The model under review builds one solid part; all positions refer to its coordinate system, in mm. A direction names the side the tool comes from. Coordinates: 2 decimals unless noted, no trailing zeros. Loops run counter-clockwise (first coordinate to the right, second up) from the corner with the lowest first, then second, coordinate; pieces in that order, holes last. Notation, with made-up numbers: M 70,67 L 97,67 A22 ccw 97,79 Z; hole C -2.75,78 d3. An arc over 180 degrees is marked long. Write item = value, one per line. Start each with the question number.
Q1. Wall thickness on probe 1 along Y at (x, z) = (-5, -3); probe 2 along Z at (x, y) = (-7.5, -3); probe 3 along Z at (x, y) = (-2, 8.75): over which ranges is each line inside the solid? List them lowest first.
Q2. Clearance check with flat-ended pins moving along their axes: pin 1 Ø4 at (x, z) = (2.5, -22) entering from -Y; pin 2 Ø8 at (y, z) = (2.5, -19.5) entering from +X; pin 3 Ø6 at (x, y) = (0.5, -7.5) entering from +Z. State where each tip first meets the part, or that it passes through.
Q3. We need section A-A on z = -14.5. Give the boundary of the cut face in (x, y), and give its area (3 significant figures).
Q4. For faces 1 (the face through (-9, 0, 0)), 2 (the face through (-9.5, 0, -15)), 3 (the face through (0, 9.5, -15)), 4 (the face through (8.11, -8.153, -14.79)), list the 3-axis set-ups (+Z, -Z, +X, -X, +Y, -Y) from which the entire face can be reached by the end or side of a thin tool; tool diameter is ignored.
from build123d import *

# Parameters (mm, degrees)
F3_DEPTH = 30


with BuildPart() as f1:
    # F0 (on Front) → F1 (revolve)
    with BuildSketch(Plane.XZ):
        with BuildLine():
            Line((11.5, 0), (8, 0))
            Line((8, 0), (8, 6.5))
            Line((8, 6.5), (11.6, 10.1))
            ThreePointArc((11.6, 10.1), (8.202439, 18.302439), (0, 21.7))
            Line((0, 21.7), (0, 0))
            Line((0, 0), (0, -30))
            Line((0, -30), (11.5, -30))
            Line((11.5, -30), (11.5, 0))
        make_face()
    revolve(axis=Axis((0, 0, 10.85), (0, 0, 1)))

    # F2 (on face) → F3 (cut)
    with BuildSketch(Plane(origin=(0, 0, -30), x_dir=(1, 0, 0), z_dir=(0, 0, -1))):
        with BuildLine():
            Line((-6.480741, 9.5), (6.480741, 9.5))
            ThreePointArc((6.480741, 9.5), (0, 11.5), (-6.480741, 9.5))
        make_face()
        with BuildLine():
            Line((9.5, 6.480741), (9.5, 0))
            Line((9.5, 0), (9.5, -6.480741))
            ThreePointArc((9.5, -6.480741), (10.98863, -3.391165), (11.5, 0))
            ThreePointArc((11.5, 0), (10.98863, 3.391165), (9.5, 6.480741))
        make_face()
        with BuildLine():
            Line((-9.5, -6.480741), (-9.5, 6.480741))
            ThreePointArc((-9.5, 6.480741), (-11.5, 0), (-9.5, -6.480741))
        make_face()
        with BuildLine():
            ThreePointArc((-6.480741, -9.5), (0, -11.5), (6.480741, -9.5))
            Line((6.480741, -9.5), (-6.480741, -9.5))
        make_face()
    extrude(amount=-F3_DEPTH, mode=Mode.SUBTRACT)


solid = f1.part
Returned:
q1.probe_1 = -9.5 to 9.5
q1.probe_2 = -30 to 0, 6.58 to 18.43
q1.probe_3 = -30 to 0, 7.48 to 17.45
q2.pin_1 = -9.5
q2.pin_2 = 9.5
q2.pin_3 = 20.78
q3.outline = M -9.5,-6.48 A11.5 ccw -6.48,-9.5 L 6.48,-9.5 A11.5 ccw 9.5,-6.48 L 9.5,6.48 A11.5 ccw 6.48,9.5 L -6.48,9.5 A11.5 ccw -9.5,6.48 Z
q3.area = 345 mm^2
q4.face_1 = none
q4.face_2 = -Z, -X, +Y, -Y
q4.face_3 = -Z, +X, -X, +Y
q4.face_4 = -Z, +X, -Y
